Autodesk Inventor part; units mm, degrees
ref_plane "YZ Plane" through (0, 0, 0) normal (1, 0, 0) x (0, 1, 0)
ref_plane "XZ Plane" through (0, 0, 0) normal (0, 1, 0) x (-1, 0, 0)
ref_plane "XY Plane" through (0, 0, 0) normal (0, 0, 1) x (1, 0, 0)
sketch "Esquisse1" plane through (0, 0, 0) normal (0, 0, 1) x (1, 0, 0)
  line L0 (0, 0) -> (400, 0)
  line L1 (400, 0) -> (400, 405)
  line L2 (400, 405) -> (0, 405)
  line L3 (0, 405) -> (0, 0)
  dimension "d0" = 400
  dimension "d1" = 405
extrude "Extrusion1" add sketch "Esquisse1" along normal blind 3
sketch "Esquisse2" plane through (0, 0, 3) normal (0, 0, 1) x (1, 0, 0)
  line L0 (5, 395) -> (250, 395)
  line L1 (250, 395) -> (250, 5)
  line L2 (250, 5) -> (5, 5)
  line L3 (5, 5) -> (5, 395)
  line L4 (0, 0) -> (400, 0)
  line L5 (0, 405) -> (0, 0)
  dimension "d4" = 390
  dimension "d5" = 5
  dimension "d6" = 5
  dimension "d7" = 245
extrude "Extrusion2" cut sketch "Esquisse2" against normal blind 3
sketch "Esquisse3" plane through (0, 0, 3) normal (0, 0, 1) x (1, 0, 0)
  line L0 (290, 230) -> (360, 230)
  line L1 (360, 230) -> (360, 206)
  line L2 (360, 206) -> (290, 206)
  line L3 (290, 206) -> (290, 230)
  line L4 (250, 395) -> (250, 5)
  line L5 (400, 405) -> (0, 405)
  circle A0 centre (300, 140) radius 10
  circle A1 centre (350, 140) radius 10
  circle A2 centre (300, 90) radius 10
  circle A3 centre (350, 90) radius 10
  line L6 (0, 0) -> (400, 0)
  dimension "d10" = 24
  dimension "d11" = 70
  dimension "d13" = 40
  dimension "d14" = 175
  dimension "d17" = 20
  dimension "d18" = 20
  dimension "d19" = 20
  dimension "d20" = 20
  dimension "d21" = 50
  dimension "d22" = 100
  dimension "d23" = 140
  dimension "d24" = 140
  dimension "d25" = 50
  dimension "d26" = 90
  dimension "d27" = 90
  dimension "d28" = 100
extrude "Extrusion3" cut sketch "Esquisse3" against normal blind 3
sketch "Esquisse4" plane through (0, 0, 3) normal (0, 0, 1) x (1, 0, 0)
  line L0 (380, 365) -> (383, 365)
  line L1 (383, 365) -> (383, 335)
  line L2 (383, 335) -> (380, 335)
  line L3 (380, 335) -> (380, 365)
  line L4 (250, 395) -> (250, 5)
  line L5 (400, 405) -> (0, 405)
  point P0 (0, 0)
  dimension "d29" = 30
  dimension "d30" = 3
  dimension "d31" = 130
  dimension "d32" = 40
extrude "Extrusion4" cut sketch "Esquisse4" against normal blind 3
sketch "Esquisse5" plane through (0, 0, 3) normal (0, 0, 1) x (1, 0, 0)
  line L0 (360, 21) -> (400, 21)
  line L1 (400, 21) -> (400, 1)
  line L2 (400, 1) -> (360, 1)
  line L3 (360, 1) -> (360, 21)
  line L4 (400, 0) -> (400, 405)
  line L5 (0, 0) -> (400, 0)
  dimension "d35" = 40
  dimension "d36" = 0
  dimension "d37" = 1
  dimension "d38" = 20
extrude "Extrusion5" cut sketch "Esquisse5" against normal blind 3
properties part number "face-avant"
Model file for the job. Use its own axes, mm. Round coordinates to 2 decimals unless told otherwise and drop trailing zeros. Write each loop counter-clockwise with the first axis right and the second up, starting at its lowest first coordinate (ties: lowest second). Pieces come first, ordered by that corner, then holes. Notation, with made-up numbers: (74.25, 42) -> (82.25, 42) arc R13 cw to (82.25, 46) -> close; hole circle Ø7 at (-10, 9.5). An arc over 180 degrees is marked (long way). Answer as CSV lines item,"result".
1. Slice it at C-C, the plane z = 2.05. List the corners of the cut face in (x, y).
Resolved:
outline,"(0, 0) -> (400, 0) -> (400, 1) -> (360, 1) -> (360, 21) -> (400, 21) -> (400, 405) -> (0, 405) -> close; hole (5, 5) -> (250, 5) -> (250, 395) -> (5, 395) -> close; hole circle Ø20 at (300, 90); hole circle Ø20 at (300, 140); hole (290, 206) -> (360, 206) -> (360, 230) -> (290, 230) -> close; hole circle Ø20 at (350, 90); hole circle Ø20 at (350, 140); hole (380, 335) -> (383, 335) -> (383, 365) -> (380, 365) -> close"
2. Pin check, flat tip, straight feed: pin 1 Ø0.9 at (y, z) = (12, 1.5) entering from +X. Stop position of the tip, or through.
Resolved:
pin 1,"x = 360"
3. Slice it at A-A, the plane x = 350. List the corners of the cut face in (y, z).
Resolved:
outline,"(0, 0) -> (80, 0) -> (80, 3) -> (0, 3) -> close; (100, 0) -> (130, 0) -> (130, 3) -> (100, 3) -> close; (150, 0) -> (206, 0) -> (206, 3) -> (150, 3) -> close; (230, 0) -> (405, 0) -> (405, 3) -> (230, 3) -> close"
4. Drill centre lines: line 1 (X direction, y = 341.5, z = 1.1); line 2 (Y direction, x = 300, z = 1.9); line 3 (X direction, y = 47, z = 1.9). Where is each one in solid material? Low to high.
Resolved:
line 1,"0 to 5, 250 to 380, 383 to 400"
line 2,"0 to 80, 100 to 130, 150 to 206, 230 to 405"
line 3,"0 to 5, 250 to 400"
5. Slice it at B-B, the plane y = 264. List the corners of the cut face in (x, z).
Resolved:
outline,"(0, 0) -> (5, 0) -> (5, 3) -> (0, 3) -> close; (250, 0) -> (400, 0) -> (400, 3) -> (250, 3) -> close"
6. Mould opens along Y. For faces 1 (the face through (318, 203, 0)), 2 (the face through (292.63, 96.76, 1.52)) say: +Y half, -Y half, draft (parallel to the pull), parting line (faces both ways), or undercut.
Resolved:
face 1,"draft"
face 2,"undercut"
7. Slice it at D-D, the plane y = 90. List the corners of the cut face in (x, z), plus the area to 3 significant figures.
Resolved:
outline,"(0, 0) -> (5, 0) -> (5, 3) -> (0, 3) -> close; (250, 0) -> (290, 0) -> (290, 3) -> (250, 3) -> close; (310, 0) -> (340, 0) -> (340, 3) -> (310, 3) -> close; (360, 0) -> (400, 0) -> (400, 3) -> (360, 3) -> close"
area,"345 mm²"
